Source: CAD feature listing. Evaluate the final solid. Frame: model axes, mm. Face numbers are marked on the shaded views. A direction names the side the tool comes from. Coordinates: 2 decimals unless noted, no trailing zeros. Loops run counter-clockwise (first coordinate to the right, second up) from the corner with the lowest first, then second, coordinate; pieces in that order, holes last.
Item 1: Section query B-B, the plane y = 47.3. Return the cut outline in (x, z), then the cut area to 3 significant figures.
Item 2: Section query D-D, the plane x = 11.5. Return the cut outline in (y, z), then the cut area to 3 significant figures.
Item 3: Section query A-A, the plane z = 10.5. Return the cut outline in (x, y).
Item 4: Line query: probe 1 along X at (y, z) = (45.7, -1.5); probe 2 along X at (y, z) = (48.3, 8); probe 3 along Y at (x, z) = (-28, 10). Output: solid intervals per line, ascending.
Item 5: Section query C-C, the plane z = -5.5. Return the cut outline in (x, y).
Item 6: Reachability of the marked faces 1, 2 and 3 from +Z, -Z, +X, -X, +Y, -Y: full face, straight path, thin tool, end or side. Return the list, or none.
Item 7: Pull-direction query (X, two-part tool) for the marked faces 4, 5 and 6; classes: +X half, -X half, draft (parallel to the pull), parting line (faces both ways), or undercut.
Item 8: Pin query (flat end, axial travel): pin 1 Ø3.5 at (x, z) = (-27.79, 8.04) entering from -Y; pin 2 Ø1.5 at (x, y) = (16.5, 45) entering from -Z; pin 3 Ø2 at (x, z) = (20.5, 7.5) entering from -Y. Return the tip coordinate at first contact, or that it passes through.
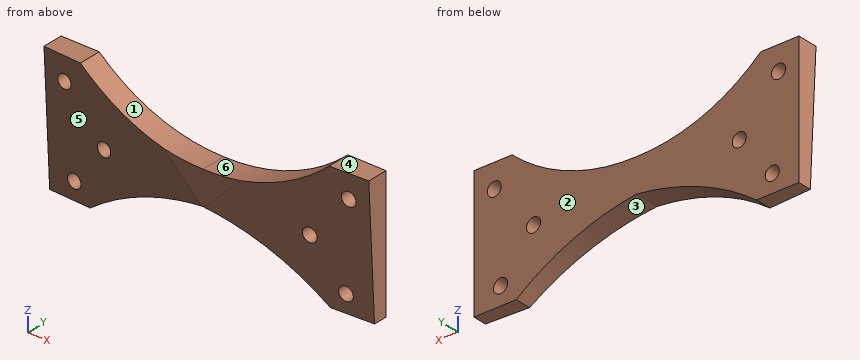
```python
from build123d import *

# Parameters (mm, degrees)
SKETCH1_W                = 31.75
SKETCH1_H                = 4.859095613
BOSS_EXTRUDE1_DEPTH      = 12.7
BOSS_EXTRUDE1_DEPTH_BACK = 12.7
SKETCH3_R                = 1.3716
CUT_EXTRUDE1_DEPTH       = 10.16


with BuildPart() as part:
    # Sketch1 → Boss-Extrude1 (new, two sides)
    with BuildSketch(Plane.XY) as boss_extrude1_sk:
        with Locations((-15.875, 46.294481234)):
            Rectangle(SKETCH1_W, SKETCH1_H)
    extrude(amount=BOSS_EXTRUDE1_DEPTH)
    extrude(boss_extrude1_sk.sketch, amount=-BOSS_EXTRUDE1_DEPTH_BACK)

    # Sketch3 → Cut-Extrude1 (cut)
    with BuildSketch(Plane(origin=(0, 48.72402904, 0), x_dir=(1, 0, 0), z_dir=(0, 1, 0))):
        with Locations(Location((-20.105647723, 0.999384842, 0), (0, 0, 180))):
            Circle(SKETCH3_R)
        with Locations(Location((-26.555704526, 9.169971692, 0), (0, 0, 180))):
            Circle(SKETCH3_R)
        with Locations(Location((-27.786476371, -8.040568412, 0), (0, 0, 180))):
            Circle(SKETCH3_R)
        with BuildLine():
            Line((0, 3.041554035), (0, 12.7))
            Line((0, 12.7), (-23.483825151, 12.7))
            ThreePointArc((-23.483825151, 12.7), (-12.393492486, 6.286506758), (0, 3.041554035))
        make_face()
        with BuildLine():
            Line((0, -3.441610433), (0, -12.7))
            Line((0, -12.7), (-24.301693504, -12.7))
            ThreePointArc((-24.301693504, -12.7), (-13.024999481, -5.776303398), (0, -3.441610433))
        make_face()
    extrude(amount=-CUT_EXTRUDE1_DEPTH, mode=Mode.SUBTRACT)

    # SurfaceCut1
    split(bisect_by=Plane(origin=(2.277212667, 43.451806158, 2.28033779), x_dir=(0.9986332910992534, -0.052192408999060975, -0.0027390420129575405), z_dir=(0.05226423163382398, 0.9972609476841369, 0.0523359562429442)), keep=Keep.TOP)

    # Mirror1: part across plane


with BuildPart() as part_1:
    add(part.part)
    add(part.part.mirror(Plane(origin=(0, 48.72402904, -12.7), x_dir=(0, 0, 1), z_dir=(-1, 0, 0))))


solid = part_1.part
```
Verdict:
1. outline: (-31.75, -12.7) - (-23.48, -12.7) arc R47.91 cw to (0, -3.04) arc R47.91 cw to (23.48, -12.7) - (31.75, -12.7) - (31.75, 12.7) - (24.3, 12.7) arc R35.66 cw to (0, 3.44) arc R35.66 cw to (-24.3, 12.7) - (-31.75, 12.7) - close; hole circle Ø2.74 at (-27.79, 8.04); hole circle Ø2.74 at (-26.56, -9.17); hole circle Ø2.74 at (-20.11, -1); hole circle Ø2.74 at (20.11, -1); hole circle Ø2.74 at (26.56, -9.17); hole circle Ø2.74 at (27.79, 8.04)
1. area: 982 mm2
2. outline: (44.02, 5.23) - (44.6, -5.93) - (48.72, -5.93) - (48.72, 5.23) - close
2. area: 49.3 mm2
3. outline: (-31.75, 44.8) - (-21.63, 44.27) - (-21.63, 48.72) - (-31.75, 48.72) - close; (21.63, 44.27) - (31.75, 44.8) - (31.75, 48.72) - (21.63, 48.72) - close
4. probe 1: x = -31.75 to -21.38, -18.83 to 18.83, 21.38 to 31.75
4. probe 2: x = -31.75 to -29.16, -26.42 to -17.78, 17.78 to 26.42, 29.16 to 31.75
4. probe 3: y = 44.63 to 48.72
5. outline: (-31.75, 45.64) - (-10.35, 44.52) - (-10.35, 48.72) - (-31.75, 48.72) - close; (10.35, 44.52) - (31.75, 45.64) - (31.75, 48.72) - (10.35, 48.72) - close
6. face 1: +Z, +Y, -Y
6. face 2: +Z, -Z, +X, -X, +Y
6. face 3: -Z, +Y, -Y
7. face 4: draft
7. face 5: -X half
7. face 6: undercut
8. pin 1: stops at y = 44.6
8. pin 2: stops at z = -8.61
8. pin 3: stops at y = 44.3
